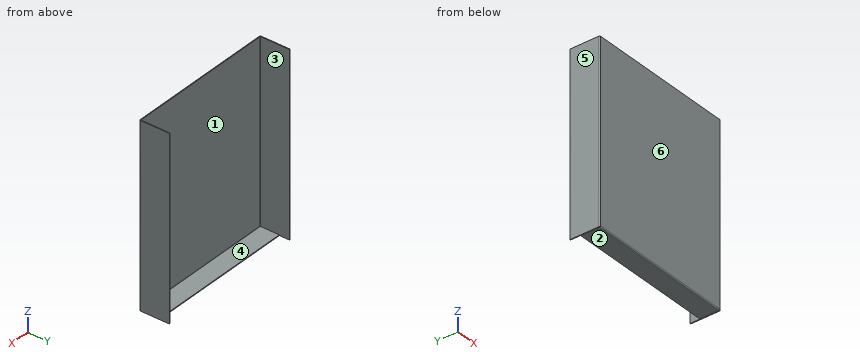
from build123d import *

# Parameters (mm, degrees)
BASE_FLANGE1_DEPTH           = 720
EDGE_FLANGE1_STRIP_W         = 14.1732
EDGE_FLANGE1_STRIP_H         = 3.175
EDGE_FLANGE1_STRIP_CUT_DEPTH = 598.5268
EDGE_FLANGE1_DEPTH           = 598.5268


# Sheet-metal steps are written as plain solids
with BuildPart() as part:
    # Sketch1 → Base-Flange1 (new body)
    with BuildSketch(Plane.XY):
        with BuildLine():
            Line((-300, 117), (-300, 0.7366))
            ThreePointArc((-300, 0.7366), (-299.784254855, 0.215745145), (-299.2634, 0))
            Line((-299.2634, 0), (299.2634, 0))
            ThreePointArc((299.2634, 0), (299.784254855, 0.215745145), (300, 0.7366))
            Line((300, 0.7366), (300, 117))
            Line((300, 117), (303.175, 117))
            Line((303.175, 117), (303.175, 0.7366))
            ThreePointArc((303.175, 0.7366), (302.029318885, -2.029318885), (299.2634, -3.175))
            Line((299.2634, -3.175), (-299.2634, -3.175))
            ThreePointArc((-299.2634, -3.175), (-302.029318885, -2.029318885), (-303.175, 0.7366))
            Line((-303.175, 0.7366), (-303.175, 117))
            Line((-303.175, 117), (-300, 117))
        make_face()
    extrude(amount=BASE_FLANGE1_DEPTH)

    # Edge-Flange1 strip (across the edge) → Edge-Flange1 strip cut (cut)
    with BuildSketch(Plane.ZY.offset(-299.2634)):
        with Locations((-3.175, -1.5875)):
            Rectangle(EDGE_FLANGE1_STRIP_W, EDGE_FLANGE1_STRIP_H)
    extrude(amount=EDGE_FLANGE1_STRIP_CUT_DEPTH, mode=Mode.SUBTRACT)

    # Edge-Flange1 section (across the edge) → Edge-Flange1 (add)
    with BuildSketch(Plane.ZY.offset(-299.2634)):
        with BuildLine():
            Line((0, 0.7366), (0, 76.825))
            Line((0, 76.825), (3.175, 76.825))
            Line((3.175, 76.825), (3.175, 0.7366))
            ThreePointArc((3.175, 0.7366), (3.390745145, 0.215745145), (3.9116, 0))
            Line((3.9116, 0), (3.9116, -3.175))
            ThreePointArc((3.9116, -3.175), (1.145681115, -2.029318885), (0, 0.7366))
        make_face()
    extrude(amount=EDGE_FLANGE1_DEPTH)


solid = part.part
The listing builds one solid part. Answer for the finished solid, in the listing's coordinates (mm). Face numbers are marked on the shaded views. A direction names the side the tool comes from. Coordinates: 2 decimals unless noted, no trailing zeros. Write each loop counter-clockwise with the first axis right and the second up, starting at its lowest first coordinate (ties: lowest second). Pieces come first, ordered by that corner, then holes. Notation, with made-up numbers: M -14,60.5 L 25,60.5 A19 ccw 25,72.5 Z; hole C 41.25,45 d2. An arc over 180 degrees is marked long. Put each result on its own line as item: value. Start each with the question number.
1. A cutting plane is placed at B-B on x = -241. Write down the section's boundary in (y, z) (3 decimals), then the cut area to 3 significant figures.
2. For a pull along X with two mould halves and no side action, classify the marked faces 4, 5 and 6 as pulls with the +X half, pulls with the -X half, needs draft (parallel to the pull), parting line crosses it, or undercut.
3. A cutting plane is placed at C-C on z = 613.5. Write down the section's boundary in (x, y) (3 decimals), then the cut area to 3 significant figures.
4. Which of the six approach directions +Z, -Z, +X, -X, +Y, -Y give full straight-line access (tool end or side, diameter ignored) to the marked faces 1, 2 and 3?
5. Flat-ended cylindrical pins translate along their axes: P1, Ø5, axis at x = 169.5, z = 484.5, coming from the +Y side; P2, Ø12, axis at x = -227.5, y = 69.5, coming from the +Z side (3 decimals); P3, Ø1, axis at y = -1.5, z = 2.5, coming from the -X side. Find the tip coordinate at first contact, or state that the pin passes through.
6. A cutting plane is placed at A-A on y = 58. Write down the section's boundary in (x, z) (3 decimals), then the cut area to 3 significant figures.
7. Consider line 1 (X direction, y = 91, z = 203.5) (3 decimals); line 2 (Y direction, x = 86, z = 392) (3 decimals); line 3 (Z direction, x = -30, y = 26) (3 decimals). Determine where each line is inside the solid, lowest interval first. Write a range as from..to.
Resolved:
1. outline: M -3.175,3.912 A3.912 ccw 0.737,0 L 76.825,0 L 76.825,3.175 L 0.737,3.175 A0.737 cw 0,3.912 L 0,720 L -3.175,720 Z
1. area: 2,530 mm2
2. face 4: undercut
2. face 5: pulls with the -X half
2. face 6: needs draft
3. outline: M -303.175,0.737 A3.912 ccw -299.263,-3.175 L 299.263,-3.175 A3.912 ccw 303.175,0.737 L 303.175,117 L 300,117 L 300,0.737 A0.737 cw 299.263,0 L -299.263,0 A0.737 cw -300,0.737 L -300,117 L -303.175,117 Z
3. area: 2,660 mm2
4. face 1: +Z, +Y
4. face 2: -Z, +X, -X, +Y, -Y
4. face 3: +Z, -Z, +Y
5. P1: stops at y = 0
5. P2: stops at z = 3.175
5. P3: stops at x = -302.77
6. outline: M -303.175,0 L -300,0 L -300,720 L -303.175,720 Z; M -299.263,0 L 299.263,0 L 299.263,3.175 L -299.263,3.175 Z; M 300,0 L 303.175,0 L 303.175,720 L 300,720 Z
6. area: 6,470 mm2
7. line 1: x = -303.175..-300, 300..303.175
7. line 2: y = -3.175..0
7. line 3: z = 0..3.175
